The model under review builds one solid part; all positions refer to its coordinate system, in mm. A direction names the side the tool comes from. Give positions to 0.01 mm unless a question says otherwise; leave off trailing zeros. Loops run counter-clockwise (first coordinate to the right, second up) from the corner with the lowest first, then second, coordinate; pieces in that order, holes last. Notation, with made-up numbers: (-15, -37.75) - (21, -37.75) arc R21 cw to (21, -20.75) - close; hole circle Ø10 at (5, 6). An arc over 180 degrees is marked (long way). Return JSON: item names as keys, results as strings. Group by question number.
from build123d import *
from build123d.topology import SkipClean

# Parameters (mm, degrees)
CROQUIS1_W                 = 15
CROQUIS1_H                 = 13
SALIENTE_EXTRUIR1_DEPTH    = 3
REDONDEO1_R                = 3
CORTAR_EXTRUIR1_DEPTH      = 63.24949799
CORTAR_EXTRUIR1_DEPTH_BACK = 63.24949799
CROQUIS2_R                 = 1.75
CORTAR_EXTRUIR2_DEPTH      = 63.24949799
CORTAR_EXTRUIR2_DEPTH_BACK = 63.24949799
CROQUIS3_R                 = 1.75
REDONDEO2_R                = 3
SALIENTE_EXTRUIR2_START    = -21
CROQUIS5_R                 = 1.75
SALIENTE_EXTRUIR2_DEPTH    = 8
SALIENTE_EXTRUIR3_START    = -29
CROQUIS6_R                 = 3
CROQUIS6_R_2               = 1.75
SALIENTE_EXTRUIR3_DEPTH    = 6


with BuildPart() as part:
    # Croquis1 → Saliente-Extruir1 (new, symmetric)
    with BuildSketch(Plane(origin=(0, 0, 0), x_dir=(1, 0, 0), z_dir=(0, 1, 0))):
        Polygon((0, 0), (0, 8), (14, 8), (14, 21), (0, 21), (0, 29), (55, 29), (55, 21), (41, 21), (41, 8), (55, 8), (55, 0), align=None)
        with Locations((27.5, 14.5)):
            Rectangle(CROQUIS1_W, CROQUIS1_H, mode=Mode.SUBTRACT)
    extrude(amount=SALIENTE_EXTRUIR1_DEPTH, both=True)

    # Redondeo1
    redondeo1_edges = [part.edges().sort_by_distance(p)[0] for p in [
        (0, -3, -4),
        (0, 3, -4),
        (0, -3, -25),
        (0, 3, -25),
        (55, -3, -4),
        (55, 3, -4),
        (55, 3, -25),
        (55, -3, -25),
    ]]
    fillet(redondeo1_edges, radius=REDONDEO1_R - 0.0001)  # a hair under: the kernel refuses the full size

    # Croquis2 → Cortar-Extruir1 (cut, two sides: drawn at the far end of the back side and taken through both)
    with BuildSketch(Plane.XY.offset(-CORTAR_EXTRUIR1_DEPTH_BACK)):
        with Locations((3, 0)):
            Circle(CROQUIS2_R)
    extrude(amount=CORTAR_EXTRUIR1_DEPTH + CORTAR_EXTRUIR1_DEPTH_BACK, mode=Mode.SUBTRACT)

    # Croquis3 → Cortar-Extruir2 (cut, two sides: drawn at the far end of the back side and taken through both)
    with BuildSketch(Plane.XY.offset(-CORTAR_EXTRUIR2_DEPTH_BACK)):
        with Locations((52, 0)):
            Circle(CROQUIS3_R)
    extrude(amount=CORTAR_EXTRUIR2_DEPTH + CORTAR_EXTRUIR2_DEPTH_BACK, mode=Mode.SUBTRACT)

    # Redondeo2
    redondeo2_edges = [part.edges().sort_by_distance(p)[0] for p in [
        (14, 0, -8),
        (14, 0, -21),
        (41, 0, -21),
        (41, 0, -8),
        (20, 0, -21),
        (20, 0, -8),
        (35, 0, -8),
        (35, 0, -21),
    ]]
    fillet(redondeo2_edges, radius=REDONDEO2_R)

    # Croquis5 → Saliente-Extruir2 (add)
    with BuildSketch(Plane.XY.offset(SALIENTE_EXTRUIR2_START)):
        with BuildLine():
            Line((0.598076211, 10.160254038), (5.598076211, 1.5))
            ThreePointArc((5.598076211, 1.5), (4.5, -2.598076211), (0.401923789, -1.5))
            Line((0.401923789, -1.5), (-4.598076211, 7.160254038))
            ThreePointArc((-4.598076211, 7.160254038), (-3.5, 11.258330249), (0.598076211, 10.160254038))
        make_face()
        with Locations(Location((-2, 8.660254038, 0), (0, 0, 180))):
            Circle(CROQUIS5_R, mode=Mode.SUBTRACT)
        with Locations((3, 0)):
            Circle(CROQUIS5_R, mode=Mode.SUBTRACT)
    extrude(amount=-SALIENTE_EXTRUIR2_DEPTH)

    # Croquis6 → Saliente-Extruir3 (add)
    with SkipClean():  # the faces are left unmerged after this step: merging them gives an invalid solid
        with BuildSketch(Plane.XY.offset(SALIENTE_EXTRUIR3_START)):
            with Locations((-2, 8.660254038)):
                Circle(CROQUIS6_R)
            with Locations((-2, 8.660254038)):
                Circle(CROQUIS6_R_2, mode=Mode.SUBTRACT)
        extrude(amount=-SALIENTE_EXTRUIR3_DEPTH)


solid = part.part
Item 1: For P1, Ø2, axis at x = 3, y = 0, coming from the +Z side; P2, Ø1.5, axis at y = 2.5, z = -28, coming from the -X side; P3, Ø6, axis at x = 11.5, z = -9, coming from the +Y side; P4, Ø1.8, axis at y = 1.5, z = -16, coming from the +X side, all flat-tipped, find the tip position at first contact; note any pin that passes through.
Item 2: Take a section at C-C (z = -5). State how many separate pieces and enclosed holes the cut face has, then the cut area to 3 significant figures.
Item 3: Tool access review of faces 1 (the face through (0.86, -2.1, -4.06)), 2 (the face through (27, 0, -8)), 3 (the face through (41.9, 0.04, -8.86)), 4 (the face through (13.14, -0.04, -20.1)): name each direction out of +Z, -Z, +X, -X, +Y, -Y from which nothing blocks a thin tool from reaching the whole face with its end or side.
Item 4: Mouldability with a two-part tool opening along Y and no side actions: class faces 5 (the face through (20.86, 0.04, -20.1)), 6 (the face through (33, 3, -21)), 7 (the face through (-2.07, 2.78, -24.94)), 8 (the face through (53.617, -0.67, -4.056)) as +Y half, -Y half, draft (parallel to the pull), parting line (faces both ways), or undercut.
Item 5: Take a section at A-A (x = 10). State the section outline as (y, z) points, then the cut area to 3 significant figures.
Item 6: Take a section at B-B (z = -13.5). State the section outline as (x, y) points, then the cut area to 3 significant figures.
Item 7: For L1, parallel to X at y = 0, z = -4; L2, parallel to Y at x = 3, z = -3.25; L3, parallel to Z at x = 7, y = -2.25, list the stretches that pass through material, from the lowest coordinate up. Write a range as from..to.
Item 8: Take a section at D-D (x = 2). State the section outline as (y, z) points.
Check sheet entries:
{
 "1": {"P1": "passes through", "P2": "stops at x = -2.34", "P3": "stops at y = 3", "P4": "stops at x = 41"},
 "2": {"separate pieces": "1", "enclosed holes": "2", "area": "303 mm^2"},
 "3": {"face 1": "+Z, -X, -Y", "face 2": "+Y, -Y", "face 3": "+X, +Y, -Y", "face 4": "-X, +Y, -Y"},
 "4": {"face 5": "draft", "face 6": "+Y half", "face 7": "-Y half", "face 8": "undercut"},
 "5": {"outline": "(-3, -29) - (3, -29) - (3, -21) - (-3, -21) - close; (-3, -8) - (3, -8) - (3, 0) - (-3, 0) - close", "area": "96.0 mm^2"},
 "6": {"outline": "(14, -3) - (20, -3) - (20, 3) - (14, 3) - close; (35, -3) - (41, -3) - (41, 3) - (35, 3) - close", "area": "72.0 mm^2"},
 "7": {"L1": "x = 0..1.25, 4.75..50.25, 53.75..55", "L2": "y = -3..-1.75, 1.75..3", "L3": "z = -29..-21, -8..0"},
 "8": {"outline": "(-2.83, -29) - (-1.44, -29) - (-1.44, -21) - (-2.83, -21) - close; (-2.83, -8) - (-1.44, -8) - (-1.44, 0) - (-2.83, 0) - close; (1.44, -29) - (7.73, -29) - (7.73, -21) - (1.44, -21) - close; (1.44, -8) - (2.83, -8) - (2.83, 0) - (1.44, 0) - close"}
}
